```python
from build123d import *

# Parameters (mm, degrees)
SKETCH003_R      = 6.064037
EXTRUDE002_DEPTH = 50
SKETCH002_W      = 78.198598
SKETCH002_H      = 41.193907
EXTRUDE001_DEPTH = 50
SKETCH001_W      = 95.175157
SKETCH001_H      = 14.36759
EXTRUDE_DEPTH    = 70
PAD_DEPTH        = 97


with BuildPart() as extrude002:
    # Sketch003 (on Face5 of Cut001) → Extrude002 (new body)
    with BuildSketch(Plane(origin=(0, 5, 0), x_dir=(-1, 0, 0), z_dir=(0, 1, 0))):
        with Locations((20.43144, 49.75)):
            Circle(SKETCH003_R)
    extrude(amount=EXTRUDE002_DEPTH)


with BuildPart() as extrude002_1:
    # Extrude002 placement: moved
    add(extrude002.part.moved(Location((0, -30, 0))))


with BuildPart() as extrude001:
    # Sketch002 (on Face26 of Cut) → Extrude001 (new body)
    with BuildSketch(Plane(origin=(0, 5, 0), x_dir=(-1, 0, 0), z_dir=(0, 1, 0))):
        with Locations((-34.130269, 48.288522)):
            Rectangle(SKETCH002_W, SKETCH002_H)
    extrude(amount=EXTRUDE001_DEPTH)


with BuildPart() as extrude001_1:
    # Extrude001 placement: moved
    add(extrude001.part.moved(Location((0, -20, 0))))


with BuildPart() as extrude_body:
    # Sketch001 (on DatumPlane) → Extrude (new body)
    with BuildSketch(Plane.XY.offset(97)):
        with Locations((43.402381, 12.183795)):
            Rectangle(SKETCH001_W, SKETCH001_H)
    extrude(amount=EXTRUDE_DEPTH)


with BuildPart() as extrude_body_1:
    # Extrude placement: moved
    add(extrude_body.part.moved(Location((0, 0, -84))))


with BuildPart() as cut002:
    # Sketch → Pad (new body)
    with BuildSketch(Plane.XY):
        Polygon((0, 0), (84.267495, 0), (84.267495, 14), (74.267495, 14), (74.267495, 9), (79.267495, 9), (79.267495, 5), (4, 5), (4, 9), (8, 9), (0, 15.213463), (0, 5), (-35, 5), (-35, 0), align=None)
    extrude(amount=PAD_DEPTH)

    # Cut: cut Extrude body
    add(extrude_body_1.part, mode=Mode.SUBTRACT)

    # Cut001: cut Extrude001
    add(extrude001_1.part, mode=Mode.SUBTRACT)

    # Cut002: cut Extrude002
    add(extrude002_1.part, mode=Mode.SUBTRACT)


solid = cut002.part
```
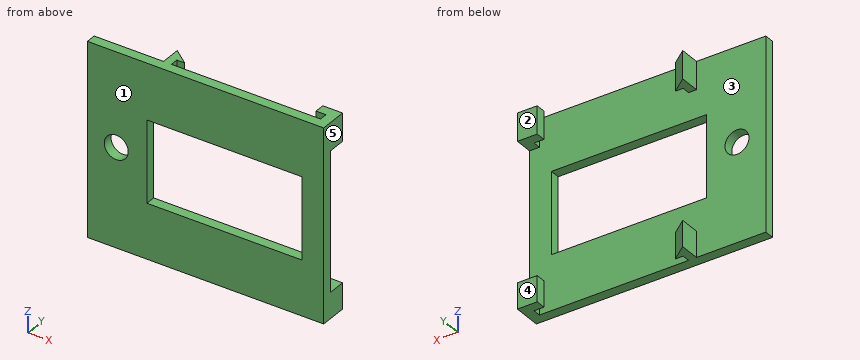
Check sheet for the modelled part. Datum: model origin and axes. Units: mm. Face numbers are marked on the shaded views. A direction names the side the tool comes from. Round coordinates to 2 decimals unless told otherwise and drop trailing zeros. Write each loop counter-clockwise with the first axis right and the second up, starting at its lowest first coordinate (ties: lowest second). Pieces come first, ordered by that corner, then holes. Notation, with made-up numbers: M -34,72.25 L -19,72.25 A23 ccw -19,108.25 Z; hole C 75,4.5 d5. An arc over 180 degrees is marked long. Write item = value, one per line. Start each with the question number.
1. Section check C-C, the plane y = 1.25. Record the cut outline in (x, z).
2. Section check D-D, the plane y = 12. Record the cut outline in (x, z).
3. Section check A-A, the plane z = 58. Record the cut outline in (x, y).
4. Gauge pin test, flat ends, axial feed: pin 1 (4.5 mm diameter, centred on x = 6, z = 89, fed in from -Y); pin 2 (12 mm diameter, centred on x = 18, z = 13, fed in from +Y); pin 3 (11 mm diameter, centred on x = -20.43, z = 49.75, fed in from +Y); pin 4 (3 mm diameter, centred on y = 9.5, z = 6, fed in from -X). Record the tip position at first contact, or that the pin passes through.
5. Tool access check on the marked faces 1 and 2. Record the directions out of +Z, -Z, +X, -X, +Y, -Y that give a thin tool (end or side, any length) a straight path to the whole face; none if there is none.
6. Section check B-B, the plane x = 30.5. Record the cut outline in (y, z).
7. Scan lines: line 1 (X direction, y = 1.6, z = 49.75); line 2 (Z direction, x = 7.5, y = 2); line 3 (Y direction, x = 11, z = 90.5). Record each from-to range of solid material in increasing order. Write a range as [from, to].
8. Release check for a two-part mould opening along X. For the marked faces 3, 4 and 5 record: pulls with the +X half, pulls with the -X half, needs draft (parallel to the pull), parting line crosses it, or undercut.
Results found:
q1.outline = M -35,0 L 84.27,0 L 84.27,97 L -35,97 Z; hole C -20.43,49.75 d12.13; hole M -4.97,27.69 L 73.23,27.69 L 73.23,68.89 L -4.97,68.89 Z
q2.outline = M 0,0 L 4.14,0 L 4.14,13 L 0,13 Z; M 0,83 L 4.14,83 L 4.14,97 L 0,97 Z; M 74.27,0 L 84.27,0 L 84.27,13 L 74.27,13 Z; M 74.27,83 L 84.27,83 L 84.27,97 L 74.27,97 Z
q3.outline = M -35,0 L -4.97,0 L -4.97,5 L -35,5 Z; M 73.23,0 L 84.27,0 L 84.27,5 L 73.23,5 Z
q4.pin_1 = 0
q4.pin_2 = 5
q4.pin_3 = through
q4.pin_4 = 0
q5.face_1 = +Z, -Z, +X, -X, -Y
q5.face_2 = +Z, -Z, +X, +Y
q6.outline = M 0,0 L 5,0 L 5,27.69 L 0,27.69 Z; M 0,68.89 L 5,68.89 L 5,97 L 0,97 Z
q7.line_1 = [-35, -26.5], [-14.37, -4.97], [73.23, 84.27]
q7.line_2 = [0, 27.69], [68.89, 97]
q7.line_3 = [0, 5]
q8.face_3 = undercut
q8.face_4 = needs draft
q8.face_5 = pulls with the +X half
